Source: CAD feature listing. Evaluate the final solid. Frame: model axes, mm. Give positions to 0.01 mm unless a question says otherwise; leave off trailing zeros. Write each loop counter-clockwise with the first axis right and the second up, starting at its lowest first coordinate (ties: lowest second). Pieces come first, ordered by that corner, then holes. Notation, with made-up numbers: M 21,63 L 47,63 A27 ccw 47,91 Z; hole C 16.25,-8.75 d6. An arc over 180 degrees is marked long. Return JSON: item names as keys, results as strings.
```python
from build123d import *

# Parameters (mm, degrees)
SKETCH1_W        = 60
SKETCH1_H        = 12
SKETCH1_W_2      = 1.5875
SKETCH1_H_2      = 3
SKETCH1_H_3      = 2
EXTRUSION1_DEPTH = 1.5875
SKETCH2_R        = 2.5
EXTRUSION2_DEPTH = 1.5875


with BuildPart() as part:
    # Sketch1 → Extrusion1 (new body)
    with BuildSketch(Plane.XY):
        with Locations((27, 5)):
            Rectangle(SKETCH1_W, SKETCH1_H)
        with Locations((-0.79375, 3.5)):
            Rectangle(SKETCH1_W_2, SKETCH1_H_2, mode=Mode.SUBTRACT)
        with Locations((-0.79375, 9)):
            Rectangle(SKETCH1_W_2, SKETCH1_H_3, mode=Mode.SUBTRACT)
        with Locations((54.79375, 9)):
            Rectangle(SKETCH1_W_2, SKETCH1_H_3, mode=Mode.SUBTRACT)
        with Locations((54.79375, 3.5)):
            Rectangle(SKETCH1_W_2, SKETCH1_H_2, mode=Mode.SUBTRACT)
    extrude(amount=EXTRUSION1_DEPTH)

    # Sketch2 → Extrusion2 (cut)
    with BuildSketch(Plane.XY.offset(1.5875)):
        with Locations((27, 7.489892181)):
            Circle(SKETCH2_R)
    extrude(amount=-EXTRUSION2_DEPTH, mode=Mode.SUBTRACT)


solid = part.part
```
1) Cut plane B-B, the plane x = 27. Return the cut outline in (y, z), then the cut area to 3 significant figures.
Numbers:
{"outline": "M -1,0 L 4.99,0 L 4.99,1.59 L -1,1.59 Z; M 9.99,0 L 11,0 L 11,1.59 L 9.99,1.59 Z", "area": "11.1 mm²"}
2) Cut plane A-A, the plane y = 3.5. Return the cut outline in (x, z), then the cut area to 3 significant figures.
Numbers:
{"outline": "M -3,0 L -1.59,0 L -1.59,1.59 L -3,1.59 Z; M 0,0 L 54,0 L 54,1.59 L 0,1.59 Z; M 55.59,0 L 57,0 L 57,1.59 L 55.59,1.59 Z", "area": "90.2 mm²"}
3) Line query: line 1 (X direction, y = 3.75, z = 1.15); line 2 (Y direction, x = 27, z = 0.85); line 3 (X direction, y = 8.75, z = 1.35). Output: solid intervals per line, ascending. Write a range as [from, to].
Numbers:
{"line 1": "x = [-3, -1.59], [0, 54], [55.59, 57]", "line 2": "y = [-1, 4.99], [9.99, 11]", "line 3": "x = [-3, -1.59], [0, 24.84], [29.16, 54], [55.59, 57]"}
4) Cut plane C-C, the plane z = 0.7. Return the cut outline in (x, y), then the cut area to 3 significant figures.
Numbers:
{"outline": "M -3,-1 L 57,-1 L 57,11 L -3,11 Z; hole M -1.59,2 L 0,2 L 0,5 L -1.59,5 Z; hole M -1.59,8 L 0,8 L 0,10 L -1.59,10 Z; hole C 27,7.49 d5; hole M 54,2 L 55.59,2 L 55.59,5 L 54,5 Z; hole M 54,8 L 55.59,8 L 55.59,10 L 54,10 Z", "area": "684 mm²"}
5) Draft query along Y for faces 1 (the face through (27, -1, 1)), 2 (the face through (27, 11, 1)), 3 (the face through (-1.588, 3, 1)), 4 (the face through (57, 5, 1)). Return one class per face: released by +Y, released by -Y, zero draft, split by the parting line, or undercut.
Numbers:
{"face 1": "released by -Y", "face 2": "released by +Y", "face 3": "undercut", "face 4": "zero draft"}
